from build123d import *

# Parameters (mm, degrees)
F0_W     = 20
F0_H     = 46
F1_DEPTH = 4
F2_D     = 5
F3_R     = 5.5
F4_DEPTH = 1.5
F5_R     = 2.5


with BuildPart() as f1:
    # F0 (on Front) → F1 (new body)
    with BuildSketch(Plane.XZ):
        Rectangle(F0_W, F0_H)
    extrude(amount=F1_DEPTH)

    # F2 (through all)
    with Locations(Plane(origin=(0, 0, 0), x_dir=(1, 0, 0), z_dir=(0, 1, 0))):
        with Locations((0, 14), (0, 0), (0, -14)):
            Hole(F2_D / 2)

    # F3 (on face) → F4 (cut)
    with BuildSketch(Plane.XZ.offset(4)):
        Circle(F3_R)
        with Locations((0, -14)):
            Circle(F3_R)
    extrude(amount=-F4_DEPTH, mode=Mode.SUBTRACT)

    # F5
    f5_edges = [f1.edges().sort_by_distance(p)[0] for p in [
        (10, -2, 23),
        (-10, -2, 23),
        (10, -2, -23),
        (-10, -2, -23),
    ]]
    fillet(f5_edges, radius=F5_R)


solid = f1.part
Read the model definition and answer for the solid it produces. Units are mm, in the model's axes. A direction names the side the tool comes from. Round coordinates to 2 decimals unless told otherwise and drop trailing zeros. Write each loop counter-clockwise with the first axis right and the second up, starting at its lowest first coordinate (ties: lowest second). Pieces come first, ordered by that corner, then holes.
1. The part is cut by section D-D, the plane z = 14. Determine the outline of the cut face in (x, y), then the cut area to 3 significant figures.
2. Determine the mould class of faces 1 (the face through (-9.287, -2.028, -22.248)), 2 (the face through (-1.19, -3.26, -5.37)), 3 (the face through (10, -2, 0)) for opening direction Z: pulls with the +Z half, pulls with the -Z half, needs draft (parallel to the pull), parting line crosses it, or undercut.
3. Given pin 1 Ø6 at (x, z) = (3.5, -1) entering from -Y; pin 2 Ø10 at (x, z) = (0, 0) entering from -Y, each flat-ended and moving along its own axis, determine where each tip first touches the part or whether it passes through.
4. The part is cut by section A-A, the plane z = 0. Determine the outline of the cut face in (x, y), then the cut area to 3 significant figures.
5. Straight lines are drawn through the part: L1, parallel to Z at x = 0, y = -0.55; L2, parallel to Z at x = 0, y = -2.9; L3, parallel to X at y = -1.55, z = 14. For each, find the intervals that lie inside material, in ascending order.
6. The part is cut by section B-B, the plane x = 1.75. Determine the outline of the cut face in (y, z), then the cut area to 3 significant figures.
7. The part is cut by section C-C, the plane y = -0.55. Determine the outline of the cut face in (x, z).
8. Which of the six approach directions +Z, -Z, +X, -X, +Y, -Y give full straight-line access (tool end or side, diameter ignored) to faces 4 (the face through (-3, -2.5, 0)), 5 (the face through (9.248, -2.028, -22.287))?
Values:
1. outline: (-10, -4) - (-2.5, -4) - (-2.5, 0) - (-10, 0) - close; (2.5, -4) - (10, -4) - (10, 0) - (2.5, 0) - close
1. area: 60.0 mm2
2. face 1: pulls with the -Z half
2. face 2: undercut
2. face 3: needs draft
3. pin 1: stops at y = -4
3. pin 2: stops at y = -2.5
4. outline: (-10, -4) - (-5.5, -4) - (-5.5, -2.5) - (-2.5, -2.5) - (-2.5, 0) - (-10, 0) - close; (2.5, -2.5) - (5.5, -2.5) - (5.5, -4) - (10, -4) - (10, 0) - (2.5, 0) - close
4. area: 51.0 mm2
5. L1: z = -23 to -16.5, -11.5 to -2.5, 2.5 to 11.5, 16.5 to 23
5. L2: z = -23 to -19.5, -8.5 to -5.5, 5.5 to 11.5, 16.5 to 23
5. L3: x = -10 to -2.5, 2.5 to 10
6. outline: (-4, -23) - (0, -23) - (0, -15.79) - (-2.5, -15.79) - (-2.5, -19.21) - (-4, -19.21) - close; (-4, -8.79) - (-2.5, -8.79) - (-2.5, -12.21) - (0, -12.21) - (0, -1.79) - (-2.5, -1.79) - (-2.5, -5.21) - (-4, -5.21) - close; (-4, 5.21) - (-2.5, 5.21) - (-2.5, 1.79) - (0, 1.79) - (0, 12.21) - (-4, 12.21) - close; (-4, 15.79) - (0, 15.79) - (0, 23) - (-4, 23) - close
6. area: 121 mm2
7. outline: (-10, -20.5) arc R2.5 ccw to (-7.5, -23) - (7.5, -23) arc R2.5 ccw to (10, -20.5) - (10, 20.5) arc R2.5 ccw to (7.5, 23) - (-7.5, 23) arc R2.5 ccw to (-10, 20.5) - close; hole circle Ø5 at (0, -14); hole circle Ø5 at (0, 0); hole circle Ø5 at (0, 14)
8. face 4: -Y
8. face 5: -Z, +X, +Y, -Y
